The listing builds one solid part. Answer for the finished solid, in the listing's coordinates (mm). A direction names the side the tool comes from. Give positions to 0.01 mm unless a question says otherwise; leave off trailing zeros. Loops run counter-clockwise (first coordinate to the right, second up) from the corner with the lowest first, then second, coordinate; pieces in that order, holes last. Notation, with made-up numbers: M -33,25 L 16,25 A17 ccw 16,39 Z; hole C 46,34.5 d1. An arc over 180 degrees is marked long. One line per item, written item: value. Start each with the question number.
Q1. For faces 5 (the flat face through (8, 55, -15.405)), 6 (the flat face through (8, 55, -28.105)), 7 (the flat face through (8, 69.469, -22)), 8 (the flat face through (8, 41.529, -22)), 9 (the cylindrical face through (0.81, 70.6, -38.06)), determine the directions among +Z, -Z, +X, -X, +Y, -Y from which every point of the face is accessible in a straight line to the end or side of a thin tool.
Q2. Flat-ended cylindrical pins translate along their axes: pin 1 (5 mm diameter, centred on y = 5.52, z = -5.25, fed in from -X); pin 2 (5 mm diameter, centred on y = 69.02, z = -5.25, fed in from +X); pin 3 (4 mm diameter, centred on x = 7.5, y = 61, fed in from +Z); pin 4 (5 mm diameter, centred on x = 12, z = -19, fed in from +Y). Find the tip coordinate at first contact, or state that the pin passes through.
Q3. A cutting plane is placed at C-C, the plane z = -38. Determine the outline of the cut face in (x, y), and give its area (3 significant figures).
Q4. A cutting plane is placed at B-B, the plane z = -17.5. Determine the outline of the cut face in (x, y).
Q5. Consider L1, parallel to Y at x = 13.25, z = -21; L2, parallel to X at y = 32, z = -37.5; L3, parallel to Z at x = 11, y = 67. Determine where each line is inside the solid, lowest interval first.
Q6. A cutting plane is placed at A-A, the plane y = 45. Determine the outline of the cut face in (x, z), and give its area (3 significant figures).
Q7. A cutting plane is placed at D-D, the plane x = 5.5. Determine the outline of the cut face in (y, z).
Q8. The mould has two halves that part along Y. Classify faces 1 (the flat face through (1, 37, 0)), 2 (the cylindrical face through (0.81, 6, -39.78)), 3 (the flat face through (1, 0, -21)), 4 (the cylindrical face through (0.81, 7.1, -5.04)): +Y half, -Y half, draft (parallel to the pull), parting line (faces both ways), or undercut.
from build123d import *

# Parameters (mm, degrees)
SKETCH1_W          = 43.5102
SKETCH1_H          = 74.549
EXTRUDE1_DEPTH     = 1.6002
SKETCH2_R          = 1.5875
CUT_EXTRUDE1_DEPTH = 2.6002
SKETCH3_W          = 12.7
SKETCH3_H          = 27.94
EXTRUDE2_DEPTH     = 12.7


with BuildPart() as part:
    # Sketch1 → Extrude1 (new body)
    with BuildSketch(Plane(origin=(0, 0, 0), x_dir=(0, 0, -1), z_dir=(1, 0, 0))):
        with Locations((21.7551, 37.2745)):
            Rectangle(SKETCH1_W, SKETCH1_H)
    extrude(amount=EXTRUDE1_DEPTH)

    # Sketch2 → Cut-Extrude1 (cut, through all)
    with BuildSketch(Plane(origin=(1.6002, 0, 0), x_dir=(0, 0, -1), z_dir=(1, 0, 0))):
        with Locations((5.2451, 69.0245)):
            Circle(SKETCH2_R)
        with Locations((38.2651, 69.0245)):
            Circle(SKETCH2_R)
        with Locations((38.2651, 5.5245)):
            Circle(SKETCH2_R)
        with Locations((5.2451, 5.5245)):
            Circle(SKETCH2_R)
    extrude(amount=-CUT_EXTRUDE1_DEPTH, mode=Mode.SUBTRACT)

    # Sketch3 → Extrude2 (add)
    with BuildSketch(Plane(origin=(1.6002, 0, 0), x_dir=(0, 0, -1), z_dir=(1, 0, 0))):
        with Locations((21.7551, 55.499)):
            Rectangle(SKETCH3_W, SKETCH3_H)
    extrude(amount=EXTRUDE2_DEPTH)


solid = part.part
Answer block:
1. face 5: +Z, +X, +Y, -Y
1. face 6: -Z, +X, +Y, -Y
1. face 7: +Z, -Z, +X, +Y
1. face 8: +Z, -Z, +X, -Y
1. face 9: +X, -X
2. pin 1: x = 0
2. pin 2: x = 1.6
2. pin 3: z = -15.41
2. pin 4: y = 69.47
3. outline: M 0,0 L 1.6,0 L 1.6,3.96 L 0,3.96 Z; M 0,7.09 L 1.6,7.09 L 1.6,67.46 L 0,67.46 Z; M 0,70.59 L 1.6,70.59 L 1.6,74.55 L 0,74.55 Z
3. area: 109 mm^2
4. outline: M 0,0 L 1.6,0 L 1.6,41.53 L 14.3,41.53 L 14.3,69.47 L 1.6,69.47 L 1.6,74.55 L 0,74.55 Z
5. L1: 41.53 to 69.47
5. L2: 0 to 1.6
5. L3: -28.11 to -15.41
6. outline: M 0,-43.51 L 1.6,-43.51 L 1.6,-28.11 L 14.3,-28.11 L 14.3,-15.41 L 1.6,-15.41 L 1.6,0 L 0,0 Z
6. area: 231 mm^2
7. outline: M 41.53,-28.11 L 69.47,-28.11 L 69.47,-15.41 L 41.53,-15.41 Z
8. face 1: draft
8. face 2: undercut
8. face 3: -Y half
8. face 4: undercut
